Could you check a few things on this drawing? It's one solid part, dimensions in mm from its lowest x, y, z. Give positions to 0.01 mm unless a question says otherwise; leave off trailing zeros. Answer as a JSON object with one key per item and string values.
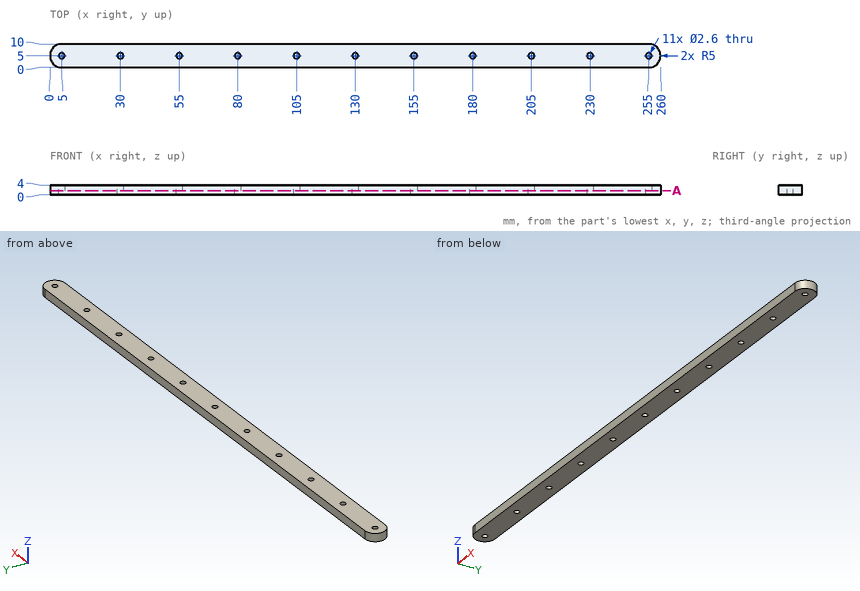
1) Imagine slicing it at A-A on z = 1.8. Give the number of separate pieces and of enclosed holes in the cut face, and give its area (3 significant figures).
Check sheet entries:
{"separate pieces": "1", "enclosed holes": "11", "area": "2,520 mm2"}
2) I'm going to push flat-ended pins straight in: P1, Ø2, axis at x = 255, y = 5, coming from the +Z side; P2, Ø3.5, axis at x = 205, y = 5, coming from the -Z side; P3, Ø2, axis at y = 3.5, z = 2.5, coming from the +X side. Where does each tip first touch, or does it pass through?
Check sheet entries:
{"P1": "through", "P2": "z = 0", "P3": "x = 259.97"}
3) I need wall thicknesses on L1, parallel to Y at x = 155, z = 2.7; L2, parallel to Y at x = 231, z = 3.1; L3, parallel to X at y = 1.75, z = 2.35. Which ranges of each line are inside material? Lowest first, please.
Check sheet entries:
{"L1": "0 to 3.7, 6.3 to 10", "L2": "0 to 4.17, 5.83 to 10", "L3": "1.2 to 258.8"}
